Geometry check sheet. Reference: the model listing, model coordinates, mm. A direction names the side the tool comes from. Give positions to 0.01 mm unless a question says otherwise; leave off trailing zeros. Write each loop counter-clockwise with the first axis right and the second up, starting at its lowest first coordinate (ties: lowest second). Pieces come first, ordered by that corner, then holes. Notation, with made-up numbers: M 67.5,27 L 77.5,27 A25 ccw 77.5,62 Z; hole C -18.5,72.5 d4. An arc over 180 degrees is marked long. One line per item, written item: value. Start each with the question number.
1. Scan lines: line 1 (Z direction, x = -19.25, y = -0.9); line 2 (X direction, y = -13, z = 7); line 3 (X direction, y = -6.5, z = 7). Record each from-to range of solid material in increasing order.
2. Cross-section at D-D on x = -67. Record the cut outline in (y, z).
3. Cross-section at C-C on z = 13.5. Record the cut outline in (x, y).
4. Release check for a two-part mould opening along Z. For faces 1 (the face through (-56, -1, 0)), 2 (the face through (-28.592, -1.014, 10.601)), 3 (the face through (-31.4, 0, 12.1)) record: pulls with the +Z half, pulls with the -Z half, needs draft (parallel to the pull), parting line crosses it, or undercut.
5. Gauge pin test, flat ends, axial feed: pin 1 (8 mm diameter, centred on y = -11, z = 16.5, fed in from +X); pin 2 (1 mm diameter, centred on y = -6.5, z = 16.5, fed in from -X); pin 3 (2 mm diameter, centred on x = -36.5, z = 17.5, fed in from -Y). Record the tip position at first contact, or that the pin passes through.
6. Cross-section at B-B on y = -14.5. Record the cut outline in (x, z).
7. Cross-section at A-A on x = -8. Record the cut outline in (y, z), then the cut area to 3 significant figures.
8. Tool access check on faces 4 (the face through (-30.4, -2, 7.6)), 5 (the face through (-82, -20, 10)). Record the directions out of +Z, -Z, +X, -X, +Y, -Y that give a thin tool (end or side, any length) a straight path to the whole face; none if there is none.
from build123d import *

# Parameters (mm, degrees)
PAD_DEPTH           = 20
SKETCH001_R         = 2
POCKET_DEPTH        = 2.001
LINEARPATTERN_COUNT = 5
LINEARPATTERN_PITCH = 11.25


with BuildPart() as part:
    # Sketch → Pad (new body)
    with BuildSketch(Plane.XY):
        with BuildLine():
            ThreePointArc((-101.908902, 0), (-81.908902, -20), (-61.908902, 0))
            Line((-61.908902, 0), (0, 0))
            Line((0, -2), (0, 0))
            Line((-60, -2), (0, -2))
            ThreePointArc((-103.908902, 0), (-82.909939, -21.977214), (-60, -2))
            Line((-103.908902, 0), (-101.908902, 0))
        make_face()
    extrude(amount=PAD_DEPTH)

    # Sketch001 → Pocket (cut, through all)
    with BuildSketch(Plane.XZ.offset(2)):
        with Locations((-53, 10)):
            Circle(SKETCH001_R)
    pocket = extrude(amount=-POCKET_DEPTH, mode=Mode.SUBTRACT)

    # LinearPattern: Pocket ×5
    with Locations(*[(i * LINEARPATTERN_PITCH, 0, 0) for i in range(1, LINEARPATTERN_COUNT)]):
        add(pocket, mode=Mode.SUBTRACT)


solid = part.part
Report:
1. line 1: z = 0 to 8, 12 to 20
1. line 2: x = -99.66 to -97.11, -66.71 to -64.16
1. line 3: x = -102.93 to -100.82, -62.99 to -60.89
2. outline: M -16.18,0 L -13.33,0 L -13.33,20 L -16.18,20 Z
3. outline: M -103.91,0 A22 ccw -60,-2 L 0,-2 L 0,0 L -61.91,0 A20 cw -101.91,0 Z
4. face 1: pulls with the -Z half
4. face 2: undercut
4. face 3: needs draft
5. pin 1: stops at x = -61.05
5. pin 2: stops at x = -103.07
5. pin 3: stops at y = -2
6. outline: M -98.45,0 L -95.68,0 L -95.68,20 L -98.45,20 Z; M -68.13,0 L -65.36,0 L -65.36,20 L -68.13,20 Z
7. outline: M -2,0 L 0,0 L 0,8 L -2,8 Z; M -2,12 L 0,12 L 0,20 L -2,20 Z
7. area: 32.0 mm^2
8. face 4: +Z, -Z, +X, -Y
8. face 5: +Z, -Z, +Y
